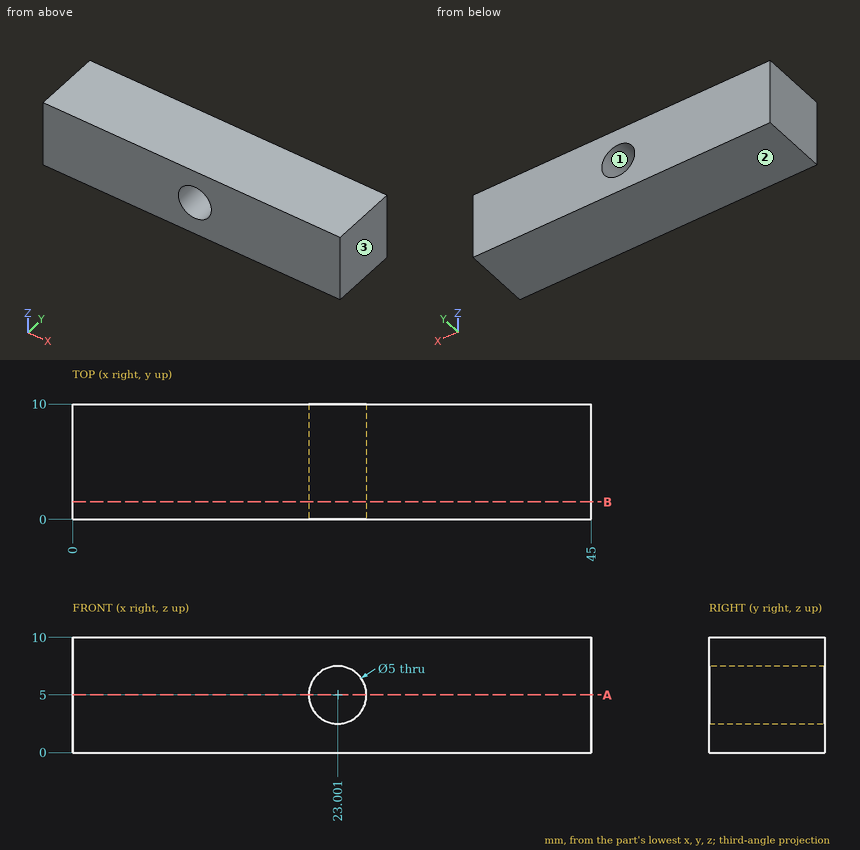
The drawing under review shows one solid part. Ordinate dimensions are in mm from its lowest x, y, z. Coordinates: 2 decimals unless noted, no trailing zeros. Write each loop counter-clockwise with the first axis right and the second up, starting at its lowest first coordinate (ties: lowest second). Pieces come first, ordered by that corner, then holes. Notation, with made-up numbers: (50, 87.25) - (75, 87.25) arc R21 ccw to (75, 98.25) - close; hole circle Ø6 at (11.25, 3.5). An arc over 180 degrees is marked (long way). Answer in a Markdown table with one row per item. Add a question column.
Q1. We need section A-A, the plane z = 5. State the section outline as (x, y) points.
Q2. Draft analysis for pull direction X (two halves, no side actions). For the marked faces 1, 2 and 3, state which applies: +X half, -X half, draft (parallel to the pull), parting line (faces both ways), or undercut.
Q3. We need section B-B, the plane y = 1.5. State the section outline as (x, z) points.
Q4. For probe 1 along X at (y, z) = (5.75, 5); probe 2 along X at (y, z) = (1, 5.5), list the stretches that pass through material, from the lowest coordinate up.
Answer list:
| question | item | result |
|---|---|---|
| 1 | outline | (0, 0) - (20.5, 0) - (20.5, 10) - (0, 10) - close; (25.5, 0) - (45, 0) - (45, 10) - (25.5, 10) - close |
| 2 | face 1 | undercut |
| 2 | face 2 | draft |
| 2 | face 3 | +X half |
| 3 | outline | (0, 0) - (45, 0) - (45, 10) - (0, 10) - close; hole circle Ø5 at (23, 5) |
| 4 | probe 1 | x = 0 to 20.5, 25.5 to 45 |
| 4 | probe 2 | x = 0 to 20.55, 25.45 to 45 |
